Could you check a few things on this model? Use its own coordinates, in mm. Face numbers are marked on the shaded views. A direction names the side the tool comes from. Give positions to 0.01 mm unless a question says otherwise; leave off trailing zeros. Write each loop counter-clockwise with the first axis right and the second up, starting at its lowest first coordinate (ties: lowest second). Pieces come first, ordered by that corner, then holes. Notation, with made-up numbers: (54, 86) - (70, 86) arc R13 cw to (70, 104) - close; hole circle Ø1 at (-19.5, -9). An arc over 180 degrees is marked (long way). Answer in a Markdown table with one row per item.
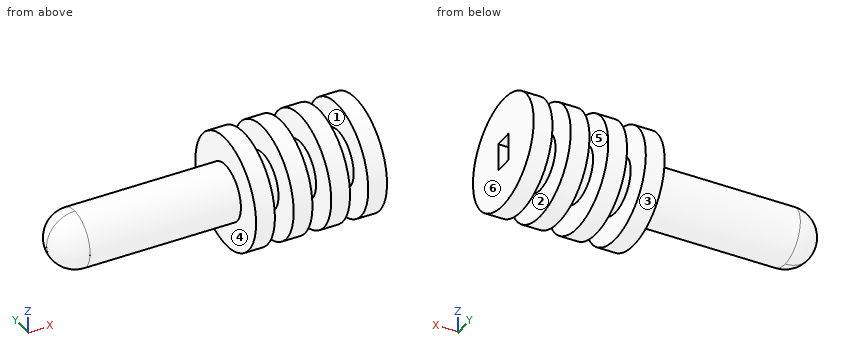
from build123d import *
from build123d import SkipClean  # not in build123d's __all__

# Parameters (mm, degrees)
F1_W     = 10
F1_H     = 15
F3_W     = 10
F3_H     = 15
F5_DEPTH = 15


with BuildPart() as f2:
    # F1 (on Front) → F2 (revolve)
    with BuildSketch(Plane.XZ):
        Polygon((150, -15), (150, 0), (140.3131330013, 0), (140, -15), align=None)
        Polygon((138.0902081728, 15), (0, 15), (0, 0), (80.3131330013, 0), (90.3131330013, 0), (100.3131330013, 0), (110.3131330013, 0), (120.3131330013, 0), (130.3131330013, 0), (140.3131330013, 0), (150, 0), (150, 15), align=None)
        with Locations((125.3131330013, -7.5)):
            Rectangle(F1_W, F1_H)
        with Locations((105.3131330013, -7.5)):
            Rectangle(F1_W, F1_H)
        with Locations((85.3131330013, -7.5)):
            Rectangle(F1_W, F1_H)
    revolve(axis=Axis((75, 0, 15), (1, 0, 0)))

    # F0 (on Front) → F4 (revolve)
    with BuildSketch(Plane.XZ):
        with BuildLine():
            ThreePointArc((0, 30), (-15, 15), (0, 0))
            Line((0, 0), (0, 30))
        make_face()
    with SkipClean():  # cleaning this boolean's faces spoils the solid; the shape is the same uncleaned
        revolve(axis=Axis((0, 0, 15), (0, 0, 1)))

    # F3 (on face) → F5 (cut)
    with BuildSketch(Plane.YZ.offset(150)):
        with Locations((0, 15)):
            Rectangle(F3_W, F3_H)
    with SkipClean():  # cleaning this boolean's faces spoils the solid; the shape is the same uncleaned
        extrude(amount=-F5_DEPTH, mode=Mode.SUBTRACT)


solid = f2.part
1) Will these pins go through, and if not, where does the flat tip stop? P1, Ø12, axis at x = 140, z = 14, coming from the +Y side; P2, Ø10, axis at x = 6, y = -16.5, coming from the +Z side; P3, Ø2, axis at y = -11, z = -7, coming from the -X side; P4, Ø11, axis at y = -2.5, z = 12.5, coming from the +X side.
Check values:
| item | result |
|---|---|
| P1 | stops at y = 30 |
| P2 | stops at z = 24.63 |
| P3 | stops at x = 80.31 |
| P4 | stops at x = 150 |
2) We'd pull the mould along Y, two halves only. Please class the marked faces 1, 2 and 3: +Y half, -Y half, draft (parallel to the pull), parting line (faces both ways), or undercut.
Check values:
| item | result |
|---|---|
| face 1 | undercut |
| face 2 | draft |
| face 3 | parting line |
3) On a 3-axis mill with a long thin cutter (end or side, diameter ignored), from which of +Z, -Z, +X, -X, +Y, -Y can I reach the whole of each face in a straight line? I mean the marked faces 4, 5 and 6. Say none if no direction works.
Check values:
| item | result |
|---|---|
| face 4 | -X |
| face 5 | none |
| face 6 | +Z, -Z, +X, +Y, -Y |
4) Imagine slicing it at B-B (x = 56.5). List the corners of the cut face in (y, z) for me, then the cut area to 3 significant figures.
Check values:
| item | result |
|---|---|
| outline | circle Ø30 at (0, 15) |
| area | 707 mm2 |
5) Imagine slicing it at A-A (z = 39). State how many separate pieces and enclosed holes the cut face has, then the cut area to 3 significant figures.
Check values:
| item | result |
|---|---|
| separate pieces | 4 |
| enclosed holes | 0 |
| area | 1,440 mm2 |
6) Imagine slicing it at D-D (x = 88). List the corners of the cut face in (y, z) for me.
Check values:
| item | result |
|---|---|
| outline | circle Ø60 at (0, 15) |
7) If I drill on line 1 (X direction, y = -6, z = -12); line 2 (X direction, y = -19.5, z = 13.5); line 3 (Z direction, x = 122.5, y = -26), over which ranges is the centre line in solid material (lowest first)?
Check values:
| item | result |
|---|---|
| line 1 | x = 80.31 to 90.31, 100.31 to 110.31, 120.31 to 130.31, 140.05 to 150 |
| line 2 | x = 80.31 to 90.31, 100.31 to 110.31, 120.31 to 130.31, 140.22 to 150 |
| line 3 | z = 0.03 to 29.97 |
